Could you check a few things on this model? Use its own coordinates, in mm. A direction names the side the tool comes from. Give positions to 0.01 mm unless a question says otherwise; leave off trailing zeros. Order: outer loops, then holes, each group sorted by start corner. A loop starts at its lowest first (then second) coordinate and runs counter-clockwise, first axis right, second up. Notation, with made-up numbers: (33.5, 43.25) -> (89.5, 43.25) arc R17 ccw to (89.5, 60.25) -> close; hole circle Ø3 at (77.5, 2). An arc over 180 degrees is marked (long way). Answer as CSV lines item,"result". Start each with the question number.
(1) I want a section at A-A (y = 2.5). Please give me the cut outline in (x, z), plus the area to 3 significant figures.
(2) We'd pull the mould along Z, two halves only. Please class faces 6 (the face through (0, 9.4, -5.3)), 7 (the face through (1, 0, 12)), 8 (the face through (0, 9, 9)): released by +Z, released by -Z, zero draft, split by the parting line, or undercut.
(3) I want a section at C-C (x = -1). Please give me the cut outline in (y, z).
(4) I need wall thicknesses on L1, parallel to X at y = 3.35, z = 13.25; L2, parallel to Z at x = -1.5, y = 1; L3, parallel to Z at x = -3.5, y = 7. Which ranges of each line are inside material? Lowest first, please.
(5) I want a section at B-B (z = 13.25). Please give me the cut outline in (x, y), plus the area to 3 significant figures.
(6) On a 3-axis mill with a long thin cutter (end or side, diameter ignored), from which of +Z, -Z, +X, -X, +Y, -Y can I reach the whole of each face in a straight line? I mean faces 1 (the face through (2.028, 9.228, -5.166)), 2 (the face through (-2.535, 9.699, 5.715)), 3 (the face through (4.493, 9.699, 5.715)), 4 (the face through (-2.217, 3.042, 11.663)), 5 (the face through (0, 9, -9)). Say none if no direction works.
(7) Will these pins go through, and if not, where does the flat tip stop? pin 1 Ø1.2 at (y, z) = (9, -5) entering from +X; pin 2 Ø5 at (x, z) = (-2, 2) entering from -Y; pin 3 Ø4 at (x, z) = (-2, -15) entering from +Y; pin 4 Ø3.5 at (x, z) = (-1, -13.25) entering from -Y.
(8) I want a section at D-D (z = -4.5). Please give me the cut outline in (x, y), plus the area to 3 significant figures.
```python
from build123d import *

# Parameters (mm, degrees)
ESBO_O1_W                      = 18.5
ESBO_O1_H                      = 13
RESSALTO_EXTRUS_O1_DEPTH       = 8
ESBO_O2_W                      = 8.5
ESBO_O2_H                      = 10
CORTE_EXTRUS_O1_DEPTH          = 21.377683872
ESBO_O3_W                      = 10
ESBO_O3_H                      = 3
RESSALTO_EXTRUS_O2_DEPTH       = 20
ESBO_O4_W                      = 10
ESBO_O4_H                      = 8
RESSALTO_EXTRUS_O3_DEPTH       = 10
ESBO_O5_W                      = 8
ESBO_O5_H                      = 3
RESSALTO_EXTRUS_O4_DEPTH       = 8.5
ESBO_O6_W                      = 5
ESBO_O6_H                      = 8
CORTE_EXTRUS_O2_DEPTH          = 22.563858653
ESBO_O7_W                      = 5
ESBO_O7_H                      = 8
CORTE_EXTRUS_O3_DEPTH          = 22.563858653
FURO_DE_DI_METRO_4_0_4_1_D     = 4
FURO_DE_DI_METRO_4_0_4_1_DEPTH = 13
FURO_DE_DI_METRO_4_0_4_2_D     = 4
FILETE1_R                      = 1
FILETE2_R                      = 2
RESSALTO_EXTRUS_O5_DEPTH       = 4
ESBO_O16_W                     = 10.570066626
ESBO_O16_H                     = 8.435311821
CORTE_EXTRUS_O4_DEPTH          = 10
ESBO_O17_W                     = 5
ESBO_O17_H                     = 6
CORTE_EXTRUS_O5_DEPTH          = 10
ESBO_O18_W                     = 5
ESBO_O18_H                     = 7.112668327
CORTE_EXTRUS_O6_DEPTH          = 22
ESBO_O19_W                     = 8.5
ESBO_O19_H                     = 3
CORTE_EXTRUS_O7_DEPTH          = 22
ESBO_O28_R                     = 2
RESSALTO_EXTRUS_O9_DEPTH       = 13
ESBO_O29_W                     = 8.5
ESBO_O29_H                     = 7
CORTE_EXTRUS_O10_DEPTH         = 25
FILETE3_R                      = 1


with BuildPart() as part:
    # Esboço1 → Ressalto-extrusão1 (new body)
    with BuildSketch(Plane(origin=(0, 0, 6), x_dir=(-1, 0, 0), z_dir=(0, 0, -1))):
        with Locations((4.25, 6.5)):
            Rectangle(ESBO_O1_W, ESBO_O1_H)
    extrude(amount=-RESSALTO_EXTRUS_O1_DEPTH)

    # Esboço2 → Corte-extrusão1 (cut, through all)
    with BuildSketch(Plane.XY.offset(14)):
        with Locations((-9.25, 8)):
            Rectangle(ESBO_O2_W, ESBO_O2_H)
    extrude(amount=-CORTE_EXTRUS_O1_DEPTH, mode=Mode.SUBTRACT)

    # Esboço3 → Ressalto-extrusão2 (add)
    with BuildSketch(Plane(origin=(0, 0, 6), x_dir=(-1, 0, 0), z_dir=(0, 0, -1))):
        with Locations((0, 11.5)):
            Rectangle(ESBO_O3_W, ESBO_O3_H)
    extrude(amount=RESSALTO_EXTRUS_O2_DEPTH)

    # Esboço4 → Ressalto-extrusão3 (add)
    with BuildSketch(Plane.XZ.offset(-10)):
        with Locations((0, -10)):
            Rectangle(ESBO_O4_W, ESBO_O4_H)
    extrude(amount=RESSALTO_EXTRUS_O3_DEPTH)

    # Esboço5 → Ressalto-extrusão4 (add)
    with BuildSketch(Plane.ZY.offset(5)):
        with Locations((-10, 1.5)):
            Rectangle(ESBO_O5_W, ESBO_O5_H)
    extrude(amount=RESSALTO_EXTRUS_O4_DEPTH)

    # Esboço6 → Corte-extrusão2 (cut, through all)
    with BuildSketch(Plane.ZY.offset(5)):
        with Locations((-11.5, 9)):
            Rectangle(ESBO_O6_W, ESBO_O6_H)
    extrude(amount=-CORTE_EXTRUS_O2_DEPTH, mode=Mode.SUBTRACT)

    # Esboço7 → Corte-extrusão3 (cut, through all)
    with BuildSketch(Plane.ZY.offset(5)):
        with Locations((11.5, 9)):
            Rectangle(ESBO_O7_W, ESBO_O7_H)
    extrude(amount=-CORTE_EXTRUS_O3_DEPTH, mode=Mode.SUBTRACT)

    # Furo de diâmetro Ø4.0 (4)1
    with Locations(Plane(origin=(0, 0, 0), x_dir=(-1, 0, 0), z_dir=(0, -1, 0))):
        with Locations((9.25, 10)):
            Hole(FURO_DE_DI_METRO_4_0_4_1_D / 2, depth=FURO_DE_DI_METRO_4_0_4_1_DEPTH)

    # Furo de diâmetro Ø4.0 (4)2 (through all)
    with Locations(Plane(origin=(0, 3, 0), x_dir=(1, 0, 0), z_dir=(0, 1, 0))):
        with Locations((-9.25, -10)):
            Hole(FURO_DE_DI_METRO_4_0_4_2_D / 2)

    # Filete1
    filete1_edges = [part.edges().sort_by_distance(p)[0] for p in [
        (0, 10, 6),
        (0, 10, -6),
        (0, 13, -9),
        (0, 5, -9),
        (0, 13, 9),
        (0, 5, 9),
    ]]
    fillet(filete1_edges, radius=FILETE1_R)

    # Filete2
    filete2_edges = [part.edges().sort_by_distance(p)[0] for p in [
        (-13.5, 1.5, 14),
        (-13.5, 1.5, 6),
        (-13.5, 1.5, -14),
        (-13.5, 1.5, -6),
    ]]
    fillet(filete2_edges, radius=FILETE2_R)

    # Esboço15 → Ressalto-extrusão5 (add)
    with BuildSketch(Plane(origin=(4, 0, 0), x_dir=(0, 0, -1), z_dir=(1, 0, 0))):
        with BuildLine():
            Line((-6, 10), (-6, 7.5))
            ThreePointArc((-6, 7.5), (-5.18496543, 9.208933408), (-3.464806021, 10))
            Line((-3.464806021, 10), (-6, 10))
        make_face()
        with BuildLine():
            ThreePointArc((3.464806021, 10), (5.18496543, 9.208933408), (6, 7.5))
            Line((6, 7.5), (6, 10))
            Line((6, 10), (3.464806021, 10))
        make_face()
    extrude(amount=-RESSALTO_EXTRUS_O5_DEPTH)

    # Esboço16 → Corte-extrusão4 (cut)
    with BuildSketch(Plane(origin=(0, 3, 0), x_dir=(1, 0, 0), z_dir=(0, 1, 0))):
        with Locations((-10.285033313, -10.21765591)):
            Rectangle(ESBO_O16_W, ESBO_O16_H)
    extrude(amount=-CORTE_EXTRUS_O4_DEPTH, mode=Mode.SUBTRACT)

    # Esboço17 → Corte-extrusão5 (cut)
    with BuildSketch(Plane(origin=(5, 0, 0), x_dir=(0, 0, -1), z_dir=(1, 0, 0))):
        with Locations((-11.5, 3)):
            Rectangle(ESBO_O17_W, ESBO_O17_H)
    extrude(amount=-CORTE_EXTRUS_O5_DEPTH, mode=Mode.SUBTRACT)

    # Esboço18 → Corte-extrusão6 (cut)
    with BuildSketch(Plane(origin=(5, 0, 0), x_dir=(0, 0, -1), z_dir=(1, 0, 0))):
        with Locations((11.5, 3.556334164)):
            Rectangle(ESBO_O18_W, ESBO_O18_H)
    extrude(amount=-CORTE_EXTRUS_O6_DEPTH, mode=Mode.SUBTRACT)

    # Esboço19 → Corte-extrusão7 (cut)
    with BuildSketch(Plane.XY.offset(-6)):
        with Locations((-9.25, 1.5)):
            Rectangle(ESBO_O19_W, ESBO_O19_H)
    extrude(amount=-CORTE_EXTRUS_O7_DEPTH, mode=Mode.SUBTRACT)

    # Esboço28 → Ressalto-extrusão9 (add, through all)
    # profile 1 of 2: a face of its own
    with BuildSketch(Plane(origin=(0, 13, 0), x_dir=(1, 0, 0), z_dir=(0, 1, 0))):
        with BuildLine():
            Line((-5, -9), (5, -9))
            Line((5, -9), (5, -15.5))
            ThreePointArc((5, -15.5), (4.414213562, -16.914213562), (3, -17.5))
            Line((3, -17.5), (-3, -17.5))
            ThreePointArc((-3, -17.5), (-4.414213562, -16.914213562), (-5, -15.5))
            Line((-5, -15.5), (-5, -9))
        make_face()
        with Locations(Location((-1, -13.25, 0), (0, 0, 270))):
            Circle(ESBO_O28_R, mode=Mode.SUBTRACT)
    # profile 2 of 2: a face of its own
    with BuildSketch(Plane(origin=(0, 13, 0), x_dir=(1, 0, 0), z_dir=(0, 1, 0))):
        with BuildLine():
            Line((3, 17.5), (-3, 17.5))
            ThreePointArc((-3, 17.5), (-4.414213562, 16.914213562), (-5, 15.5))
            Line((-5, 15.5), (-5, 9))
            Line((-5, 9), (5, 9))
            Line((5, 9), (5, 15.5))
            ThreePointArc((5, 15.5), (4.414213562, 16.914213562), (3, 17.5))
        make_face()
        with Locations(Location((-1, 13.25, 0), (0, 0, 90))):
            Circle(ESBO_O28_R, mode=Mode.SUBTRACT)
    extrude(amount=-RESSALTO_EXTRUS_O9_DEPTH)

    # Esboço29 → Corte-extrusão10 (cut)
    with BuildSketch(Plane.ZY.offset(5)):
        with Locations((-13.25, 9.5)):
            Rectangle(ESBO_O29_W, ESBO_O29_H)
        with Locations((13.25, 9.5)):
            Rectangle(ESBO_O29_W, ESBO_O29_H)
    extrude(amount=-CORTE_EXTRUS_O10_DEPTH, mode=Mode.SUBTRACT)

    # Filete3
    filete3_edges = [part.edges().sort_by_distance(p)[0] for p in [
        (0, 6, -9),
        (0, 6, 9),
    ]]
    fillet(filete3_edges, radius=FILETE3_R)


solid = part.part
```
Final values:
1,outline,"(-5, -15.5) arc R2 ccw to (-3, -17.5) -> (3, -17.5) arc R2 ccw to (5, -15.5) -> (5, -6) -> (-5, -6) -> close; (-5, 6) -> (5, 6) -> (5, 15.5) arc R2 ccw to (3, 17.5) -> (-3, 17.5) arc R2 ccw to (-5, 15.5) -> close; hole circle Ø4 at (-1, -13.25); hole circle Ø4 at (-1, 13.25)"
1,area,"201 mm²"
2,face 6,"undercut"
2,face 7,"zero draft"
2,face 8,"released by +Z"
3,outline,"(0, -17.5) -> (6, -17.5) -> (6, -15.25) -> (0, -15.25) -> close; (0, -11.25) -> (6, -11.25) -> (6, -10) arc R1 cw to (7, -9) -> (12, -9) arc R1 ccw to (13, -8) -> (13, 8) arc R1 ccw to (12, 9) -> (7, 9) arc R1 cw to (6, 10) -> (6, 11.25) -> (0, 11.25) -> (0, 6) -> (9, 6) arc R1 cw to (10, 5) -> (10, -5) arc R1 cw to (9, -6) -> (0, -6) -> close; (0, 15.25) -> (6, 15.25) -> (6, 17.5) -> (0, 17.5) -> close"
4,L1,"-5 to -3, 1 to 5"
4,L2,"-17.5 to -15.19, -11.31 to -6, 6 to 11.31, 15.19 to 17.5"
4,L3,"-9 to -6, 6 to 9"
5,outline,"(-5, 0) -> (-3, 0) -> (-3, 6) -> (-5, 6) -> close; (1, 0) -> (5, 0) -> (5, 6) -> (1, 6) -> close"
5,area,"36.0 mm²"
6,face 1,"+X, -X, -Y"
6,face 2,"-X, -Y"
6,face 3,"+X, -Y"
6,face 4,"+Y, -Y"
6,face 5,"-Z, +X, -X, +Y"
7,pin 1,"x = 4"
7,pin 2,"y = 10"
7,pin 3,"y = 6"
7,pin 4,"through"
8,outline,"(-5, 10) -> (0, 10) -> (0, 9.7) -> (4, 9.7) -> (4, 10) -> (5, 10) -> (5, 13) -> (-5, 13) -> close"
8,area,"31.2 mm²"
